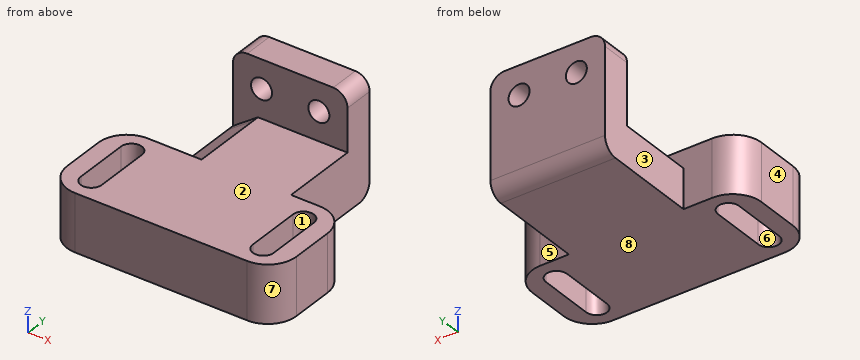
Autodesk Inventor part; units mm, degrees
ref_plane "YZ Plane" through (0, 0, 0) normal (1, 0, 0) x (0, 1, 0)
ref_plane "XZ Plane" through (0, 0, 0) normal (0, 1, 0) x (-1, 0, 0)
ref_plane "XY Plane" through (0, 0, 0) normal (0, 0, 1) x (1, 0, 0)
sketch "Sketch1" plane through (0, 0, 0) normal (0, 0, 1) x (1, 0, 0)
  line L0 (-19.1352, -8.5102) -> (-19.1352, 8.3898) construction
  line L1 (-16.8111, -6.1861) -> (-16.8111, 6.0657)
  line L2 (-21.4593, 6.0657) -> (-21.4593, -6.1861)
  arc A0 (-21.4593, -6.1861) -> (-16.8111, -6.1861) centre (-19.1352, -6.1861) ccw
  arc A1 (-16.8111, 6.0657) -> (-21.4593, 6.0657) centre (-19.1352, 6.0657) ccw
  line L3 (18.9648, -8.5102) -> (18.9648, 8.3898) construction
  line L4 (21.2889, -6.1861) -> (21.2889, 6.0657)
  line L5 (16.6407, 6.0657) -> (16.6407, -6.1861)
  arc A2 (16.6407, -6.1861) -> (21.2889, -6.1861) centre (18.9648, -6.1861) ccw
  arc A3 (21.2889, 6.0657) -> (16.6407, 6.0657) centre (18.9648, 6.0657) ccw
  line L6 (-19.1352, 8.3898) -> (18.9648, 8.3898)
  line L7 (18.9648, -8.5102) -> (-19.1352, -8.5102)
  line L8 (25.3148, 11.0523) -> (-25.4852, 11.0523)
  line L9 (-25.4852, 11.0523) -> (-25.4852, -11.1727)
  line L10 (-25.4852, -11.1727) -> (25.3148, -11.1727)
  line L11 (25.3148, -11.1727) -> (25.3148, 11.0523)
  line L12 (25.3148, 11.0523) -> (-25.4852, -11.1727) construction
  line L13 (-25.4852, 11.0523) -> (25.3148, -11.1727) construction
  point P0 (0, 0)
  point P1 (-0.0852, -0.0602)
  point P2 (-19.1352, -0.0602)
  point P3 (18.9648, -0.0602)
  dimension "d0" = 4.6482
  dimension "d1" = 4.6482
  dimension "d2" = 50.8
  dimension "d3" = 22.225
extrude "Extrusion1" add sketch "Sketch1" along normal blind 12.7 contours L1 A1 L6 A3 L5 A2 L7 A0 | L11 L10 L9 L8
sketch "Sketch2" plane through (-25.4852, 11.0523, 0) normal (0, 1, 0) x (1, 0, 0)
  line L0 (0, 0) -> (50.8, 0)
  line L1 (0, 0) -> (12.7, 0)
  line L2 (12.7, 0) -> (12.7, -12.7)
  line L3 (12.7, -12.7) -> (0, -12.7)
  line L4 (0, -12.7) -> (0, 0)
  line L5 (50.8073, 0) -> (38.1073, 0)
  line L6 (38.1073, 0) -> (38.1073, -12.7)
  line L7 (38.1073, -12.7) -> (50.8073, -12.7)
  line L8 (50.8, 0) -> (50.8, -12.7)
  line L9 (50.8, 0) -> (50.8, -12.7)
  line L10 (50.8, -12.7) -> (50.8, 0)
  line L11 (50.8, 0) -> (38.1073, 0)
  point P0 (25.4852, 0)
  dimension "d7" = 12.7
  dimension "d8" = 12.7
  dimension "d9" = 12.7
  dimension "d10" = 12.7
extrude "Extrusion2" add sketch "Sketch2" along normal blind 22.3933
chamfer "Chamfer1" distance 3.9688 distance2 5.5563 1 edges at (12.6221, 22.2489, 12.7) measured on face at (12.6221, 18.5167, 4.2333)
chamfer "Chamfer2" distance 4.7625 distance2 7.9375 1 edges at (-12.7852, 22.2489, 0) measured on face at (-12.7852, 18.5167, 8.4667)
sketch "Sketch3" plane through (-25.4852, 33.4456, 0) normal (0, 1, 0) x (1, 0, 0)
  line L0 (0, 0) -> (6.319, 0)
  line L1 (38.1073, 0) -> (4.7625, 0)
  line L2 (6.319, -0.6519) -> (0, -0.6519)
  line L3 (0, 0) -> (0, -12.7)
  line L4 (0, 0) -> (0, -0.6519)
  line L5 (6.319, 0) -> (6.319, -0.6519)
  point P0 (25.4852, 0)
extrude "Extrusion3" cut sketch "Sketch3" against normal up to surface (22.3933 mm away)
fillet "Fillet2" radius 3.175 2 edges at (-19.6363, 22.2489, 0.6519) (-25.4852, 22.2489, 0.6519)
sketch "Sketch4" plane through (0, 0, 12.7) normal (0, 0, 1) x (1, 0, 0)
  line L0 (-12.7852, 11.0523) -> (-18.8822, 11.0523)
  line L1 (-12.7852, 11.0523) -> (-12.7852, 26.6987)
  line L2 (-12.7852, 33.4456) -> (-12.7852, 11.0523)
  line L3 (-12.7852, 11.0523) -> (25.3148, 11.0523)
  line L4 (25.3148, -11.1727) -> (25.3148, 33.4456)
  line L5 (25.3148, 11.0523) -> (25.3148, 26.6987)
  line L6 (12.6221, 33.4456) -> (12.6221, 11.0523)
  line L7 (-25.4852, -11.1727) -> (-25.4852, 33.4456)
  line L8 (25.3148, 26.6987) -> (12.6221, 26.6987)
  line L9 (12.6221, 26.6987) -> (12.6221, 36.2237)
  line L10 (25.3148, 36.2237) -> (25.3148, 26.6987)
  line L11 (-12.7852, 26.6987) -> (-25.4852, 26.6987)
  line L12 (-25.4852, 26.6987) -> (-25.4852, 36.2237)
  line L13 (-12.7852, 36.2237) -> (-12.7852, 26.6987)
  line L14 (18.1783, 33.4456) -> (12.6221, 33.4456)
  line L15 (25.3148, 33.4456) -> (12.6221, 33.4456)
  line L16 (-12.7852, 36.2237) -> (-12.7852, 33.4456)
  line L17 (-25.4852, 33.4456) -> (-12.7852, 33.4456)
  line L18 (-12.7852, 33.4456) -> (-25.4852, 33.4456)
  line L19 (-25.4852, 33.4456) -> (-25.4852, 36.2237)
  line L20 (12.6221, 33.4456) -> (12.6221, 26.6987)
  line L21 (25.3148, 26.6987) -> (25.3148, 33.4456)
  line L22 (-12.7852, 26.6987) -> (-12.7852, 33.4456)
  line L23 (-25.4852, 26.6987) -> (-25.4852, 33.4456)
  point P0 (0, 0)
  dimension "d22" = 15.6464
extrude "Extrusion4" add sketch "Sketch4" along normal blind 12.7 contours L2 L11 L7 L17 | L6 L14 L15 L4 L8
extrude "Extrusion5" add sketch "Sketch4" against normal blind 4.2333 contours L6 L14 L15 L4 L8
sketch "Sketch5" plane through (-25.4852, 33.4456, 0) normal (0, 1, 0) x (1, 0, 0)
  line L0 (50.8, -25.4) -> (38.1073, -25.4)
  line L1 (12.7, -25.4) -> (0, -25.4)
  line L2 (44.4537, -25.4) -> (44.4537, -19.05)
  line L3 (6.35, -25.4) -> (6.35, -19.05)
  circle A0 centre (6.35, -19.05) radius 2.3241
  circle A1 centre (44.4537, -19.05) radius 2.3241
  point P0 (25.4852, 0)
  dimension "d27" = 6.35
  dimension "d28" = 6.35
  dimension "d29" = 4.6482
  dimension "d30" = 4.6482
extrude "Extrusion6" cut sketch "Sketch5" against normal through all
sketch "Sketch6" plane through (-12.7852, 11.0523, 12.7) normal (1, 0, 0) x (0, 0, -1)
  line L0 (-12.7, 15.6464) -> (-12.7, 22.3933)
  line L1 (0, 15.6464) -> (-12.7, 15.6464)
  line L2 (-12.7, 15.6464) -> (-12.7, 22.3933)
  line L3 (-12.7, 22.3933) -> (0, 22.3933)
  line L4 (0, 22.3933) -> (0, 15.6464)
  line L5 (0, 15.6464) -> (-12.7, 15.6464)
  point P0 (12.7, -11.0523)
extrude "Extrusion7" [suppressed]
sketch "Sketch7" plane through (18.1783, 26.6987, 12.7) normal (0, -1, 0) x (1, 0, 0)
  circle A0 centre (-37.3136, 6.35) radius 2.3241
  circle A1 centre (0.7901, 6.35) radius 2.3241
  line L0 (-37.3136, 6.35) -> (-24.6136, 6.35)
  line L1 (-24.6136, 6.35) -> (-11.9136, 6.35)
  line L2 (-26.798, 4.1656) -> (-22.4292, 4.1656)
  line L3 (-22.4292, 4.1656) -> (-22.4292, 8.5344)
  line L4 (-22.4292, 8.5344) -> (-26.798, 8.5344)
  line L5 (-26.798, 8.5344) -> (-26.798, 4.1656)
  line L6 (-26.798, 4.1656) -> (-22.4292, 8.5344) construction
  line L7 (-22.4292, 4.1656) -> (-26.798, 8.5344) construction
  line L8 (-9.7292, 8.5344) -> (-14.098, 8.5344)
  line L9 (-9.7292, 4.1656) -> (-9.7292, 8.5344)
  line L10 (-14.098, 4.1656) -> (-9.7292, 4.1656)
  line L11 (-14.098, 8.5344) -> (-14.098, 4.1656)
  point P0 (-18.1783, -12.7)
  dimension "d35" = 12.7
  dimension "d36" = 12.7
  dimension "d37" = 4.3688
  dimension "d38" = 4.3688
  dimension "d41" = 12.7
extrude "Extrusion8" [suppressed]
fillet "Fillet3" [suppressed]
sketch "Sketch8" plane through (-25.4852, 11.0523, 0) normal (0, 1, 0) x (1, 0, 0)
  line L0 (38.1073, 0) -> (0, 0)
  line L1 (0, 0) -> (14.6548, 0)
  line L2 (14.6548, 0) -> (14.6548, -26.951)
  line L3 (14.6548, -26.951) -> (0, -26.951)
  line L4 (0, -26.951) -> (0, 0)
  point P0 (25.4852, 0)
  point P1 (14.6548, 0)
extrude "Extrusion9" cut sketch "Sketch8" along normal blind 25.4
sketch "Sketch9" plane through (25.3148, -11.1727, 12.7) normal (1, 0, 0) x (0, 0, -1)
  line L0 (0, 0) -> (0, 37.8714)
  line L1 (12.7, 0) -> (0, 0)
  line L2 (12.7, 0) -> (12.7, 44.6183)
  line L3 (12.7, 44.6183) -> (-12.7, 44.6183)
  line L4 (-12.7, 37.8714) -> (-12.7, 44.6183)
  line L5 (0, 37.8714) -> (-12.7, 37.8714)
  point P0 (12.7, 11.1727)
extrude "Extrusion10" add sketch "Sketch9" along normal blind 12.7
sketch "Sketch10" plane through (-25.4852, 33.4456, 0) normal (0, 1, 0) x (1, 0, 0)
  circle A0 centre (44.4537, -19.05) radius 2.3241
  line L0 (44.4537, -19.05) -> (57.1537, -19.05)
  circle A1 centre (57.1537, -19.05) radius 2.3241
  point P0 (25.4852, 0)
  dimension "d58" = 12.7
  dimension "d59" = 4.6482
extrude "Extrusion11" cut sketch "Sketch10" against normal blind 12.7 contours A1
fillet "Fillet9" radius 3.175 2 edges at (12.6221, 30.0721, 25.4) (38.0148, 30.0721, 25.4)
fillet "Fillet10" radius 6.35 3 edges at (-25.4852, 11.0523, 6.35) (-25.4852, -11.1727, 6.35) (38.0148, -11.1727, 6.35)
sketch "Sketch11" plane through (-25.4852, 33.4456, 0) normal (0, 1, 0) x (1, 0, 0)
  arc A0 (60.325, -25.4) -> (63.5, -22.225) centre (60.325, -22.225) ccw
  line L0 (63.5, 0) -> (63.5, -22.225)
  line L1 (38.1073, 0) -> (63.5, 0)
  line L2 (38.1073, 0) -> (38.1073, -22.225)
  arc A1 (38.1073, -22.225) -> (41.2823, -25.4) centre (41.2823, -22.225) ccw
  line L3 (41.2823, -25.4) -> (60.325, -25.4)
  circle A2 centre (57.1537, -19.05) radius 2.3241
  circle A3 centre (44.4537, -19.05) radius 2.3241
  point P0 (25.4852, 0)
extrude "Extrusion12" add sketch "Sketch11" along normal blind 1.5875
sketch "Sketch12" plane through (18.1783, 26.6987, 12.7) normal (0, -1, 0) x (1, 0, 0)
  circle A0 centre (13.4901, 6.35) radius 2.3241
  circle A1 centre (0.7901, 6.35) radius 2.3241
  arc A2 (19.8364, 9.525) -> (16.6614, 12.7) centre (16.6614, 9.525) ccw
  line L0 (-2.3813, 12.7) -> (16.6614, 12.7)
  arc A3 (-2.3813, 12.7) -> (-5.5563, 9.525) centre (-2.3813, 9.525) ccw
  line L1 (-5.5563, -3.9688) -> (-5.5563, 9.525)
  line L2 (0, 0) -> (-5.5563, -3.9688)
  line L3 (19.8364, 0) -> (0, 0)
  line L4 (19.8364, 9.525) -> (19.8364, 0)
  point P0 (-18.1783, -12.7)
extrude "Extrusion13" cut sketch "Sketch12" against normal blind 1.5875
fillet "Fillet12" radius 3.175 1 edges at (25.3184, 35.0331, 0)
sketch "Sketch13" plane through (0, 0, 12.7) normal (0, 0, 1) x (1, 0, 0)
  arc A0 (31.6648, -11.1727) -> (38.0148, -4.8227) centre (31.6648, -4.8227) ccw
  line L0 (38.0148, 28.2862) -> (38.0148, -4.8227)
  line L1 (38.0148, 28.2862) -> (18.1783, 28.2862)
  line L2 (18.1783, 11.0523) -> (18.1783, 28.2862)
  line L3 (18.1783, 11.0523) -> (-19.1352, 11.0523)
  arc A1 (-19.1352, 11.0523) -> (-25.4852, 4.7023) centre (-19.1352, 4.7023) ccw
  line L4 (-25.4852, -4.8227) -> (-25.4852, 4.7023)
  arc A2 (-25.4852, -4.8227) -> (-19.1352, -11.1727) centre (-19.1352, -4.8227) ccw
  line L5 (-19.1352, -11.1727) -> (31.6648, -11.1727)
  arc A3 (16.6407, -6.1861) -> (21.2889, -6.1861) centre (18.9648, -6.1861) ccw
  line L6 (16.6407, -6.1861) -> (16.6407, 6.0657)
  arc A4 (21.2889, 6.0657) -> (16.6407, 6.0657) centre (18.9648, 6.0657) ccw
  line L7 (21.2889, 6.0657) -> (21.2889, -6.1861)
  arc A5 (-21.4593, -6.1861) -> (-16.8111, -6.1861) centre (-19.1352, -6.1861) ccw
  line L8 (-21.4593, -6.1861) -> (-21.4593, 6.0657)
  arc A6 (-16.8111, 6.0657) -> (-21.4593, 6.0657) centre (-19.1352, 6.0657) ccw
  line L9 (-16.8111, 6.0657) -> (-16.8111, -6.1861)
  line L10 (-19.1352, 6.0657) -> (-19.1352, -6.1861) construction
  line L11 (-21.4593, 6.0657) -> (-21.4593, -6.1861)
  line L12 (-16.8111, -6.1861) -> (-16.8111, 6.0657)
  arc A7 (-16.8111, 6.0657) -> (-21.4593, 6.0657) centre (-19.1352, 6.0657) ccw
  arc A8 (-21.4593, -6.1861) -> (-16.8111, -6.1861) centre (-19.1352, -6.1861) ccw
  line L13 (-19.1352, -0.0602) -> (-18.0483, -0.0602)
  arc A9 (8.5889, 6.0657) -> (3.9407, 6.0657) centre (6.2648, 6.0657) ccw
  line L14 (8.5889, -6.1861) -> (8.5889, 6.0657)
  line L15 (3.9407, 6.0657) -> (3.9407, -6.1861)
  arc A10 (3.9407, -6.1861) -> (8.5889, -6.1861) centre (6.2648, -6.1861) ccw
  arc A11 (46.6889, 6.0657) -> (42.0407, 6.0657) centre (44.3648, 6.0657) ccw
  line L16 (46.6889, -6.1861) -> (46.6889, 6.0657)
  arc A12 (42.0407, -6.1861) -> (46.6889, -6.1861) centre (44.3648, -6.1861) ccw
  line L17 (42.0407, 6.0657) -> (42.0407, -6.1861)
  line L18 (18.9648, -0.0602) -> (20.0517, -0.0602)
  line L19 (-25.4852, 4.7023) -> (-25.4852, -4.8227)
  line L20 (-25.4852, -4.8227) -> (-25.4852, 4.7023)
  arc A13 (-19.1352, 11.0523) -> (-25.4852, 4.7023) centre (-19.1352, 4.7023) ccw
  arc A14 (-25.4852, -4.8227) -> (-19.1352, -11.1727) centre (-19.1352, -4.8227) ccw
  arc A15 (6.2648, 11.0523) -> (-0.0852, 4.7023) centre (6.2648, 4.7023) ccw
  line L21 (-0.0852, -4.8227) -> (-0.0852, 4.7023)
  arc A16 (-0.0852, -4.8227) -> (6.2648, -11.1727) centre (6.2648, -4.8227) ccw
  line L22 (6.2648, -0.0602) -> (25.3148, -0.0602)
  line L23 (25.3148, -0.0602) -> (25.3148, 2.455)
  arc A17 (50.7148, 4.7023) -> (44.3648, 11.0523) centre (44.3648, 4.7023) ccw
  line L24 (50.7148, -4.8227) -> (50.7148, 4.7023)
  arc A18 (44.3648, -11.1727) -> (50.7148, -4.8227) centre (44.3648, -4.8227) ccw
  line L25 (6.2648, 11.0523) -> (44.3648, 11.0523)
  line L26 (44.3648, -11.1727) -> (6.2648, -11.1727)
  point P0 (0, 0)
  point P1 (6.2648, 11.0523)
  point P2 (6.2648, -11.1727)
  point P3 (38.0148, 11.0523)
  point P4 (31.6648, -11.1727)
  dimension "d73" = 25.4
  dimension "d80" = 38.1
  dimension "d87" = 25.4
  dimension "d92" = 19.05
extrude "Extrusion14" cut sketch "Sketch13" against normal blind 25.4 contours L5 A2 L4 A1 L3 A15 L21 A16 | L14 A10 L15 A9
extrude "Extrusion15" add sketch "Sketch13" against normal up to surface (12.7 mm away) contours A0 L0 L25 A17 L24 A18 L26 | L6 L22 L18 L7 A3 | L6 A4 L7 L22 L18
properties part number "Optical Mount 24"
Can you work these out from the model? Positions are in its coordinate system, mm. Face numbers are marked on the shaded views. A direction names the side the tool comes from. Give positions to 0.01 mm unless a question says otherwise; leave off trailing zeros. Loops run counter-clockwise (first coordinate to the right, second up) from the corner with the lowest first, then second, coordinate; pieces in that order, holes last. Notation, with made-up numbers: (3, 45) -> (7, 45) arc R12 ccw to (7, 54) -> close; hole circle Ø6 at (57.25, 45). An arc over 180 degrees is marked (long way). Use one line per item in the form item = value.
1) Will these pins go through, and if not, where does the flat tip stop? pin 1 (5 mm diameter, centred on y = 24.5, z = 11.5, fed in from +X); pin 2 (4 mm diameter, centred on x = 31, z = 18, fed in from -Y); pin 3 (1.5 mm diameter, centred on x = 19.5, y = 6, fed in from +Z); pin 4 (3 mm diameter, centred on x = 28, z = 13.5, fed in from -Y).
Answers:
pin_1 = 38.01
pin_2 = 28.29
pin_3 = 12.7
pin_4 = -11.17
2) If we section it at D-D (y = 7): Please give me the cut outline in (x, z).
Answers:
outline = (0.35, 0) -> (4.14, 0) -> (4.14, 12.7) -> (0.35, 12.7) -> close; (8.39, 0) -> (42.24, 0) -> (42.24, 12.7) -> (8.39, 12.7) -> close; (46.49, 0) -> (50.28, 0) -> (50.28, 12.7) -> (46.49, 12.7) -> close
3) If we section it at C-C (x = 28): Please give me the cut outline in (y, z) (3 decimals), plus the area to 3 significant figures.
Answers:
outline = (-11.173, 0) -> (31.858, 0) arc R3.175 ccw to (35.033, 3.175) -> (35.033, 25.4) -> (28.286, 25.4) -> (28.286, 12.7) -> (-11.173, 12.7) -> close
area = 670 mm²
4) I need wall thicknesses on line 1 along X through (y, z) = (31.75, 19.05); line 2 along X through (y, z) = (-2, 4); line 3 along Y through (x, z) = (44.5, 8.25). Which ranges of each line are inside material? Lowest first, please.
Answers:
line_1 = 12.62 to 16.64, 21.29 to 29.34, 33.99 to 38.01
line_2 = -0.09 to 3.94, 8.59 to 42.04, 46.69 to 50.71
line_3 = -11.17 to -8.51, 8.39 to 11.05
5) We'd pull the mould along Y, two halves only. Please class the marked faces 6, 7 and 8: released by +Y, released by -Y, zero draft, split by the parting line, or undercut.
Answers:
face_6 = undercut
face_7 = released by -Y
face_8 = zero draft
6) For the marked faces 1, 2, 3, 4 and 5, which set-ups out of +Z, -Z, +X, -X, +Y, -Y let a thin tool reach every point of the face, with its end or its side?
Answers:
face_1 = +Z, -Z
face_2 = +Z, +X, -X, -Y
face_3 = +Z, -Z, -X, +Y
face_4 = +Z, -Z, -X, +Y, -Y
face_5 = +Z, -Z, +X, +Y
7) If we section it at B-B (z = 17.5): Please give me the cut outline in (x, y).
Answers:
outline = (12.62, 28.29) -> (17.24, 28.29) -> (17.24, 35.03) -> (12.62, 35.03) -> close; (20.7, 28.29) -> (29.94, 28.29) -> (29.94, 35.03) -> (20.7, 35.03) -> close; (33.4, 28.29) -> (38.01, 28.29) -> (38.01, 35.03) -> (33.4, 35.03) -> close
8) If we section it at A-A (z = 5.5): Please give me the cut outline in (x, y).
Answers:
outline = (-0.09, -4.82) arc R6.35 ccw to (6.26, -11.17) -> (44.36, -11.17) arc R6.35 ccw to (50.71, -4.82) -> (50.71, 4.7) arc R6.35 ccw to (44.36, 11.05) -> (38.01, 11.05) -> (38.01, 35.03) -> (12.62, 35.03) -> (12.62, 11.05) -> (6.26, 11.05) arc R6.35 ccw to (-0.09, 4.7) -> close; hole (3.94, -6.19) arc R2.32 ccw to (8.59, -6.19) -> (8.59, 6.07) arc R2.32 ccw to (3.94, 6.07) -> close; hole (42.04, -6.19) arc R2.32 ccw to (46.69, -6.19) -> (46.69, 6.07) arc R2.32 ccw to (42.04, 6.07) -> close
